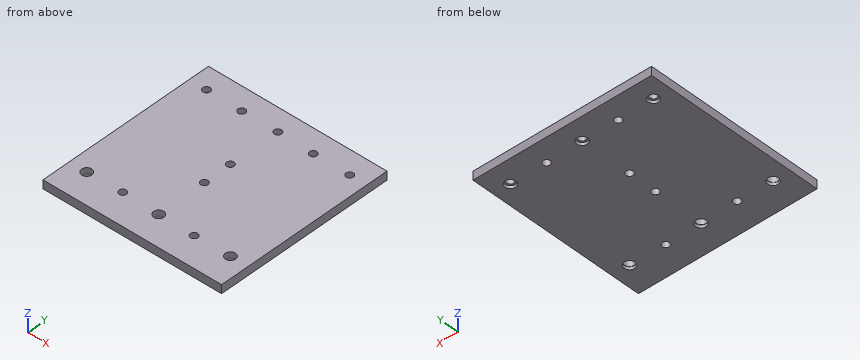
Autodesk Inventor part; units mm, degrees
ref_plane "YZ Plane" through (0, 0, 0) normal (1, 0, 0) x (0, 1, 0)
ref_plane "XZ Plane" through (0, 0, 0) normal (0, 1, 0) x (-1, 0, 0)
ref_plane "XY Plane" through (0, 0, 0) normal (0, 0, 1) x (1, 0, 0)
ref_plane "Work Plane1" through (0, 0, 0) normal (0, 0, 1) x (1, 0, 0)
sketch "Sketch1" plane through (0, 0, 0) normal (0, 0, 1) x (1, 0, 0)
  line L0 (-62.5, -65) -> (-62.5, 60.2)
  line L1 (62.5, -65) -> (-62.5, -65)
  line L2 (-62.5, 60.2) -> (62.5, 60.2)
  line L3 (62.5, 60.2) -> (62.5, -65)
  circle A0 centre (50.2, 45) radius 2.55
  circle A1 centre (50.2, -45) radius 3.55
  circle A2 centre (-50.2, -45) radius 2.55
  circle A3 centre (-50.2, 45) radius 2.55
  line L4 (-50.2, -87.1872) -> (-50.2, 86.9163) construction
  line L5 (0, -90.5792) -> (0, 86.9163) construction
  line L6 (50.2, -82.9351) -> (50.2, 98.888) construction
  line L7 (-25.1, -100.0293) -> (-25.1, 98.888) construction
  line L8 (25.1, -87.1872) -> (25.1, 98.888) construction
  line L9 (-84.1215, -10) -> (86.0151, -10) construction
  line L10 (-84.1215, 10) -> (86.0151, 10) construction
  point P0 (0, 0)
  point P1 (0, 45)
  point P2 (0, -45)
  point P3 (-25.1, -45)
  point P4 (25.1, -45)
  point P5 (25.1, 45)
  point P6 (-25.1, 45)
  point P7 (0, 0)
  point P8 (0, -10)
  point P9 (0, 10)
  dimension "d0" = 100.4
  dimension "d1" = 50.2
  dimension "d2" = 25.1
  dimension "d3" = 25.1
  dimension "d4" = 10
  dimension "d5" = 20
extrude "Extrusion1" add sketch "Sketch1" along normal blind 6 contours L0 L2 L3 L1 | A0 | A1 | A2 | A3
sketch "Sketch2" plane through (0, 0, 0) normal (0, 0, -1) x (-1, 0, 0)
  point P0 (0, 0)
  point P1 (-50.176, -44.9419)
  point P2 (-0.1594, -45.1078)
  point P3 (50.2816, -45.0688)
hole "Hole1" at (50.176, -44.9419, 0) at (0.1594, -45.1078, 0) at (-50.2816, -45.0688, 0) direction (0, 0, 1) diameter 7.1 end through all counterbore diameter 7.5 counterbore depth 2
sketch "Sketch3" plane through (0, 0, 0) normal (0, 0, -1) x (-1, 0, 0)
  point P0 (0, 0)
  point P1 (50.3086, 45.5821)
  point P2 (0.2433, 45.4506)
  point P3 (-50.5722, 44.8972)
hole "Hole2" at (-50.3086, 45.5821, 0) at (-0.2433, 45.4506, 0) at (50.5722, 44.8972, 0) direction (0, 0, 1) diameter 5.1 end through all counterbore diameter 7.5 counterbore depth 2
sketch "Sketch4" plane through (0, 0, 0) normal (0, 0, -1) x (-1, 0, 0)
  point P0 (0, 0)
  point P1 (25.3396, 45.2378)
  point P2 (-25.1139, 44.8345)
  point P3 (-25.1745, -45.3838)
  point P4 (25.6326, -44.5055)
  point P5 (0.0949, -10.3157)
  point P6 (0.3775, 9.6536)
hole "Hole3" at (25.1139, 44.8345, 0) at (-25.3396, 45.2378, 0) at (25.1745, -45.3838, 0) at (-25.6326, -44.5055, 0) at (-0.0949, -10.3157, 0) at (-0.3775, 9.6536, 0) direction (0, 0, 1) diameter 5.1 end through all
sketch "Sketch5" plane through (0, 0, 6) normal (0, 0, 1) x (1, 0, 0)
  line L0 (54.8683, -25.7428) -> (1.0212, -25.7428) construction
  line L1 (1.0212, -25.7428) -> (1.0212, -17.8731) construction
  line L2 (1.0212, -17.8731) -> (54.8683, -17.8731) construction
  line L3 (54.8683, -17.8731) -> (54.8683, -25.7428) construction
  point P0 (0, 0)
equation "\"d1\" = 0.5 * d0"
equation "\"d2\" = 0.5 * d1"
equation "\"d3\" = d2"
properties part number "X axis carriage small 2"
Build history of the part. All positions in model axes, mm. Coordinates: 2 decimals unless noted, no trailing zeros. Order: outer loops, then holes, each group sorted by start corner. A loop starts at its lowest first (then second) coordinate and runs counter-clockwise, first axis right, second up. Notation, with made-up numbers: (54, 26.5) - (78, 26.5) arc R27 ccw to (78, 58.5) - close; hole circle Ø4 at (59, 14). An arc over 180 degrees is marked (long way). Write item = value, one per line. Start each with the question number.
1) Saw through at A-A on y = 9.5. Write the cut outline in (x, z), then the cut area to 3 significant figures.
2) Flat gauge pins, fed straight in: pin 1 Ø4 at (x, y) = (50.5, 44) entering from -Z; pin 2 Ø6.5 at (x, y) = (-50.28, -45.07) entering from +Z. Where does each tip first touch, or does it go through?
3) Saw through at B-B on z = 3.7. Count the separate pieces of the cut face and the enclosed holes in it, then the cut area to 3 significant figures.
4) Wall check: line 1 along Y through (x, z) = (52, 5); line 2 along X through (y, z) = (-11, 0.8). Give the ranges that are in metal, low to high. Write a range as from..to.
From the geometry:
q1.outline = (-62.5, 0) - (-2.92, 0) - (-2.92, 6) - (-62.5, 6) - close; (2.17, 0) - (62.5, 0) - (62.5, 6) - (2.17, 6) - close
q1.area = 719 mm^2
q2.pin_1 = 2
q2.pin_2 = through
q3.separate_pieces = 1
q3.enclosed_holes = 12
q3.area = 15,300 mm^2
q4.line_1 = -65..-47.99, -41.9..42.78, 47.01..60.2
q4.line_2 = -62.5..-2.55, 2.36..62.5
